Could you check a few things on this model? Use its own coordinates, in mm. A direction names the side the tool comes from. Give positions to 0.01 mm unless a question says otherwise; leave off trailing zeros. Order: outer loops, then holes, each group sorted by start corner. A loop starts at its lowest first (then second) coordinate and runs counter-clockwise, first axis right, second up. Notation, with made-up numbers: (84, 54.25) -> (119, 54.25) arc R19 ccw to (119, 74.25) -> close; hole circle Ø7 at (-5.75, 63.25). An arc over 180 degrees is marked (long way). One line per item, written item: value.
```python
from build123d import *

# Parameters (mm, degrees)
SKETCH_2_R           = 5
EXTRUDE_1_DEPTH      = 3.75
SKETCH_3_R           = 3.525
EXTRUDE_2_DEPTH      = 4
EXTRUDE_START        = 24
SKETCH_4_R           = 3.525
EXTRUDE_3_DEPTH      = 24
CUT_EXTRUDE_START    = 5.15
SKETCH_5_OUTSIDE_W   = 18.952
SKETCH_5_OUTSIDE_H   = 18.952
SKETCH_5_OUTSIDE_W_2 = 12.787470862
SKETCH_5_OUTSIDE_H_2 = 5
CUT_EXTRUDE_1_DEPTH  = 19.08
SKETCH_6_R           = 1.19
CUT_EXTRUDE_2_DEPTH  = 8
SKETCH_7_R           = 1.475
CUT_EXTRUDE_3_DEPTH  = 1.5
SKETCH_8_OUTSIDE_W   = 18.952
SKETCH_8_OUTSIDE_H   = 18.952
SKETCH_8_OUTSIDE_R   = 3.495
CUT_EXTRUDE_5_DEPTH  = 18.85


with BuildPart() as part:
    # 草图2 → 凸台-拉伸1 (new body)
    with BuildSketch(Plane(origin=(0, 0, 0), x_dir=(0, 0, -1), z_dir=(1, 0, 0))):
        Circle(SKETCH_2_R)
    extrude(amount=EXTRUDE_1_DEPTH)

    # 草图3 → 凸台-拉伸2 (add)
    with BuildSketch(Plane.ZY):
        Circle(SKETCH_3_R)
    extrude(amount=EXTRUDE_2_DEPTH)

    # 草图4 → 凸台-拉伸3 (add)
    with BuildSketch(Plane(origin=(3.75, 0, 0), x_dir=(0, 0, -1), z_dir=(1, 0, 0)).offset(EXTRUDE_START)):
        with Locations(Location((0, 0, 0), (0, 0, 180))):
            Circle(SKETCH_4_R)
    extrude(amount=-EXTRUDE_3_DEPTH)

    # 草图5 outside → 切除-拉伸1 (cut)
    with BuildSketch(Plane(origin=(3.75, 0, 0), x_dir=(0, 0, -1), z_dir=(1, 0, 0)).offset(CUT_EXTRUDE_START)):
        Rectangle(SKETCH_5_OUTSIDE_W, SKETCH_5_OUTSIDE_H)
        Rectangle(SKETCH_5_OUTSIDE_W_2, SKETCH_5_OUTSIDE_H_2, mode=Mode.SUBTRACT)
    extrude(amount=CUT_EXTRUDE_1_DEPTH, mode=Mode.SUBTRACT)

    # 草图6 → 切除-拉伸2 (cut)
    with BuildSketch(Plane(origin=(27.75, 0, 0), x_dir=(0, 0, -1), z_dir=(1, 0, 0))):
        Circle(SKETCH_6_R)
    extrude(amount=-CUT_EXTRUDE_2_DEPTH, mode=Mode.SUBTRACT)

    # 草图7 → 切除-拉伸3 (cut)
    with BuildSketch(Plane(origin=(27.75, 0, 0), x_dir=(0, 0, -1), z_dir=(1, 0, 0))):
        Circle(SKETCH_7_R)
    extrude(amount=-CUT_EXTRUDE_3_DEPTH, mode=Mode.SUBTRACT)

    # 草图8 outside → 切除-拉伸5 (cut)
    with BuildSketch(Plane(origin=(27.75, 0, 0), x_dir=(0, 0, -1), z_dir=(1, 0, 0))):
        Rectangle(SKETCH_8_OUTSIDE_W, SKETCH_8_OUTSIDE_H)
        Circle(SKETCH_8_OUTSIDE_R, mode=Mode.SUBTRACT)
    extrude(amount=-CUT_EXTRUDE_5_DEPTH, mode=Mode.SUBTRACT)


solid = part.part
```
1) For P1, Ø1.9, axis at y = 0, z = 0, coming from the +X side; P2, Ø2, axis at y = 1, z = -1, coming from the +X side; P3, Ø2.5, axis at x = 23, z = -1, coming from the -Y side; P4, Ø5.5, axis at x = 20, z = 0.5, coming from the +Y side, each with a flat end and sliding along its axis, tell me the tip position at first contact or that it passes through.
Answer below:
P1: stops at x = 19.75
P2: stops at x = 27.75
P3: stops at y = -2.5
P4: stops at y = 2.5
2) Suppose I cut it at B-B, the plane x = 23. Write out the boundary of the cut face in (y, z) (3 decimals).
Answer below:
outline: (-2.5, -2.442) arc R3.495 ccw to (2.5, -2.442) -> (2.5, 2.442) arc R3.495 ccw to (-2.5, 2.442) -> close; hole circle Ø2.38 at (0, 0)
3) We'd pull the mould along Y, two halves only. Please class faces 4 (the cylindrical face through (27.01, 0.065, 1.474)), 5 (the cylindrical face through (18.457, 0.039, 3.495)), 6 (the flat face through (18, -2.5, 0)): +Y half, -Y half, draft (parallel to the pull), parting line (faces both ways), or undercut.
Answer below:
face 4: undercut
face 5: parting line
face 6: -Y half
4) Suppose I cut it at A-A, the plane z = 0. Write out the boundary of the cut face in (x, y) (3 decimals), then the cut area to 3 significant figures.
Answer below:
outline: (-4, -3.525) -> (0, -3.525) -> (0, -5) -> (3.75, -5) -> (3.75, -3.525) -> (8.9, -3.525) -> (8.9, -2.5) -> (27.75, -2.5) -> (27.75, -1.475) -> (26.25, -1.475) -> (26.25, -1.19) -> (19.75, -1.19) -> (19.75, 1.19) -> (26.25, 1.19) -> (26.25, 1.475) -> (27.75, 1.475) -> (27.75, 2.5) -> (8.9, 2.5) -> (8.9, 3.525) -> (3.75, 3.525) -> (3.75, 5) -> (0, 5) -> (0, 3.525) -> (-4, 3.525) -> close
area: 176 mm2
5) For faces 1 (the flat face through (0, -3.3, -2.2)), 2 (the flat face through (18, 2.5, 0)), 3 (the cylindrical face through (6.361, 3.441, -0.764)), which set-ups out of +Z, -Z, +X, -X, +Y, -Y let a thin tool reach every point of the face, with its end or its side?
Answer below:
face 1: -X
face 2: +Z, -Z, +X, +Y
face 3: +X
6) If I drill on line 1 along Y through (x, z) = (27.05, 0) (3 decimals); line 2 along Y through (x, z) = (22.5, 0); line 3 along Y through (x, z) = (13, -0.25), over which ranges is the centre line in solid material (lowest first)?
Answer below:
line 1: y = -2.5 to -1.475, 1.475 to 2.5
line 2: y = -2.5 to -1.19, 1.19 to 2.5
line 3: y = -2.5 to 2.5
7) Suppose I cut it at C-C, the plane y = 0. Write out the boundary of the cut face in (x, z) (3 decimals), then the cut area to 3 significant figures.
Answer below:
outline: (-4, -3.525) -> (0, -3.525) -> (0, -5) -> (3.75, -5) -> (3.75, -3.525) -> (8.9, -3.525) -> (8.9, -3.495) -> (27.75, -3.495) -> (27.75, -1.475) -> (26.25, -1.475) -> (26.25, -1.19) -> (19.75, -1.19) -> (19.75, 1.19) -> (26.25, 1.19) -> (26.25, 1.475) -> (27.75, 1.475) -> (27.75, 3.495) -> (8.9, 3.495) -> (8.9, 3.525) -> (3.75, 3.525) -> (3.75, 5) -> (0, 5) -> (0, 3.525) -> (-4, 3.525) -> close
area: 214 mm2
8) Suppose I cut it at D-D, the plane x = 7. Write out the boundary of the cut face in (y, z) (3 decimals).
Answer below:
outline: circle Ø7.05 at (0, 0)
